CAD build for the part. Positions are in the model's coordinates, mm. Face numbers are marked on the shaded views. Coordinates: 2 decimals unless noted, no trailing zeros. Write each loop counter-clockwise with the first axis right and the second up, starting at its lowest first coordinate (ties: lowest second). Pieces come first, ordered by that corner, then holes. Notation, with made-up numbers: (72, 27) - (81, 27) arc R27 ccw to (81, 61) - close; hole circle Ø9 at (86.25, 1). An arc over 180 degrees is marked (long way). One line per question, with ' | ' between items. Start each with the question number.
1. Band-saw the part on C-C, the plane y = 0.5. Write the cut outline in (x, z).
2. Probe line 1 (X direction, y = 2, z = -13); line 2 (X direction, y = -2, z = -13.75); line 3 (Y direction, x = 6, z = 0.5). List the from-to ranges inside material, lowest first.
3. Flat gauge pins, fed straight in: P1, Ø1.6, axis at x = 1.5, y = 1.5, coming from the -Z side; P2, Ø8, axis at x = 4, z = -10.5, coming from the -Y side; P3, Ø1, axis at x = -5, y = 0, coming from the -Z side; P4, Ø0.8, axis at x = -6, y = -2, coming from the -Z side. Where does each tip first touch, or does it go through?
4. Band-saw the part on D-D, the plane y = -1.5. Write the cut outline in (x, z).
5. Band-saw the part on A-A, the plane z = -10.25. Write the cut outline in (x, y), then the cut area to 3 significant figures.
6. Band-saw the part on B-B, the plane x = -6. Write the cut outline in (y, z).
7. Two-plate mould, pull along Y, no slides. Class the marked faces 1, 2 and 3: +Y half, -Y half, draft (parallel to the pull), parting line (faces both ways), or undercut.
from build123d import *

# Parameters (mm, degrees)
BOSS_EXTRUDE1_DEPTH = 6
CUT_EXTRUDE1_REACH  = 33.573
CHAMFER2_SIZE       = 0.5


with BuildPart() as part:
    # Sweep3: sweep along a path in Sketch1
    with BuildLine(Plane(origin=(0, 0, 0), x_dir=(1, 0, 0), z_dir=(0, 1, 0))) as sweep3_path:
        Line((-20, 21), (-20, 4))
        ThreePointArc((-20, 4), (-18.828427125, 1.171572875), (-16, 0))
        Line((-16, 0), (16, 0))
        ThreePointArc((16, 0), (18.828427125, 1.171572875), (20, 4))
        Line((20, 4), (20, 21))
    # Sketch2 → Sweep3 (sweep)
    with BuildSketch(Plane.XY.offset(-21)):
        Polygon((18.2, 1), (18.2, 3), (22.8, 3), (22.8, -3), (17, -3), (17, -1), (20.8, -1), (20.8, 1), align=None)
    sweep(path=sweep3_path.line)

    # Sketch5 → Boss-Extrude1 (add, through all)
    with BuildSketch(Plane.XZ.offset(3)):
        Polygon((-16, 2.8), (-18.816652224, 2.8), (-20.808326112, 0.808326112), align=None)
    boss_extrude1 = extrude(amount=-BOSS_EXTRUDE1_DEPTH)

    # Mirror2: Boss-Extrude1 across plane
    add(boss_extrude1.mirror(Plane(origin=(0, 0, 0), x_dir=(0, 0, 1), z_dir=(1, 0, 0))))

    # Sketch6 → Cut-Extrude1 (cut, up to next)
    with BuildSketch(Plane(origin=(0, 3, 0), x_dir=(1, 0, 0), z_dir=(0, 1, 0)), mode=Mode.PRIVATE) as cut_extrude1_sk1:
        with BuildLine():
            Line((-8, 0.3), (8, 0.3))
            ThreePointArc((8, 0.3), (9.060660172, 0.49375696), (9.984313483, 1.05))
            ThreePointArc((9.984313483, 1.05), (10.907966795, 1.60624304), (11.968626967, 1.8))
            Line((11.968626967, 1.8), (-11.968626967, 1.8))
            ThreePointArc((-11.968626967, 1.8), (-10.907966795, 1.60624304), (-9.984313483, 1.05))
            ThreePointArc((-9.984313483, 1.05), (-9.060660172, 0.49375696), (-8, 0.3))
        make_face()
    cut_extrude1_tool1 = extrude(cut_extrude1_sk1.sketch, amount=-CUT_EXTRUDE1_REACH, mode=Mode.PRIVATE) & part.part
    add(cut_extrude1_tool1.solids().sort_by_distance((0, 3, -1.083194))[0], mode=Mode.SUBTRACT)

    # Chamfer2
    chamfer2_edges = [part.edges().sort_by_distance(p)[0] for p in [
        (13.984313483, 3, -1.8),
        (-10.907966795, 3, -1.60624304),
        (-9.060660172, 3, -0.49375696),
        (0, 3, -0.3),
        (9.060660172, 3, -0.49375696),
        (10.907966795, 3, -1.60624304),
        (0, -3, -3),
        (0, -3, 2.8),
        (0, 3, 2.8),
        (-13.984313483, 3, -1.8),
        (16.707106781, -3, -3.292893219),
        (17.555634919, 3, -2.444365081),
        (17, -3, -12.5),
        (19.9, -3, -21),
        (22.8, -3, -12.5),
        (22.8, 3, -12.5),
        (20.5, 3, -21),
        (18.2, 3, -12.5),
        (-17, -3, -12.5),
        (-22.8, -3, -12.5),
        (-22.8, 3, -12.5),
        (-18.2, 3, -12.5),
        (-16.707106781, -3, -3.292893219),
        (-22.282380821, -3, -1.39775266),
        (-19.812489168, 3, 1.804163056),
        (0, 3, 2.8),
        (0, -3, 2.8),
        (-19.812489168, -3, 1.804163056),
        (-22.282380821, 3, -1.39775266),
        (-17.555634919, 3, -2.444365081),
        (22.282380821, 3, -1.39775266),
        (22.282380821, -3, -1.39775266),
        (0, -3, 2.8),
        (19.812489168, -3, 1.804163056),
        (19.812489168, 3, 1.804163056),
        (0, 3, 2.8),
    ]]
    chamfer(chamfer2_edges, length=CHAMFER2_SIZE)

    # Sketch4 for Loft1 → Loft1 section 0
    with BuildSketch(Plane.ZY.offset(-20.8)):
        with BuildLine():
            Line((-21, -1), (-13, -1))
            # circular arc as an exact rational Bezier (weights 1, cos(half-angle), 1)
            Bezier((-13, -1), (-17, -0.899984373), (-21, -1), weights=[1, 0.999687549, 1])
        make_face()
    # Sketch3 for Loft1 → Loft1 section 1
    with BuildSketch(Plane.ZY.offset(-17)):
        with BuildLine():
            Line((-21, -1), (-13, -1))
            Bezier((-13, -1), (-17, -0.396605908), (-21, -1), weights=[1, 0.988812927, 1])
        make_face()
    loft1 = loft()

    # Mirror1: Loft1 across plane
    add(loft1.mirror(Plane(origin=(0, 0, 0), x_dir=(0, 0, 1), z_dir=(1, 0, 0))))


solid = part.part
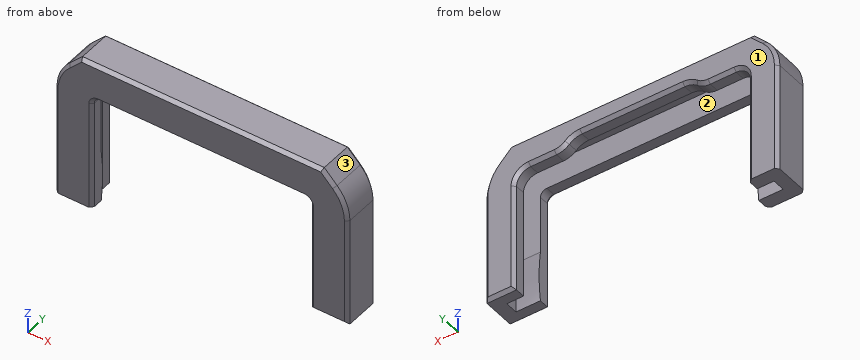
Filled in:
1) outline: (-22.8, -21) - (-20.8, -21) - (-20.8, -4) arc R4.8 cw to (-16, 0.8) - (16, 0.8) arc R4.8 cw to (20.8, -4) - (20.8, -21) - (22.8, -21) - (22.8, -4) arc R6.8 ccw to (20.81, 0.81) - (18.82, 2.8) - (-18.82, 2.8) - (-20.81, 0.81) arc R6.8 ccw to (-22.8, -4) - close
2) line 1: x = -22.8 to -18.2, 18.2 to 22.8 | line 2: x = -22.8 to -17, 17 to 22.8 | line 3: y = -3 to -1, 1 to 3
3) P1: stops at z = -0.3 | P2: passes through | P3: stops at z = 0.8 | P4: stops at z = -3
4) outline: (-22.8, -21) - (-17, -21) - (-17, -4) arc R1 cw to (-16, -3) - (16, -3) arc R1 cw to (17, -4) - (17, -21) - (22.8, -21) - (22.8, -4) arc R6.8 ccw to (20.81, 0.81) - (18.82, 2.8) - (-18.82, 2.8) - (-20.81, 0.81) arc R6.8 ccw to (-22.8, -4) - close
5) outline: (-22.8, -2.5) - (-22.3, -3) - (-17.5, -3) - (-17, -2.5) - (-17, -1) - (-20.8, -1) - (-20.8, 1) - (-18.2, 1) - (-18.2, 2.5) - (-18.7, 3) - (-22.3, 3) - (-22.8, 2.5) - close; (17, -2.5) - (17.5, -3) - (22.3, -3) - (22.8, -2.5) - (22.8, 2.5) - (22.3, 3) - (18.7, 3) - (18.2, 2.5) - (18.2, 1) - (20.8, 1) - (20.8, -1) - (17, -1) - close | area: 48.6 mm²
6) outline: (-3, -2.5) - (-2.5, -3) - (-1, -3) - (-1, 0.8) - (1, 0.8) - (1, -0.3) - (2.5, -0.3) - (3, 0.2) - (3, 2.3) - (2.5, 2.8) - (-2.5, 2.8) - (-3, 2.3) - close
7) face 1: +Y half | face 2: undercut | face 3: draft
